Autodesk Fusion 360 part; units mm, degrees
sketch "草图1" plane through (0, 0, 0) normal (0, 1, 0) x (1, 0, 0)
  circle A0 centre (0, 0) radius 10
  circle A1 centre (0, 0) radius 8
  dimension "d1" = 2
extrude "拉伸1" add sketch "草图1" along normal blind 3 contours A1 makes body 1
extrude "拉伸2" add sketch "草图1" along normal blind 5 separate body makes body 2
cylinder "圆柱体基本要素1" add diameter 2 height 20 placed x (1, 0, 0) y (0, 0, -1) z (0, 1, 0) at (20, 0, 1) separate body makes body 3
move_body "对齐1" bodies 3 to x (1, 0, 0) y (0, 1, 0) z (0, 0, 1) at (-20, 0, -1)
pattern_linear "R-阵列1" count 2 spacing 6 along (0, 0, 1) count 2 spacing 4 along (1, 0, 0) of bodies 3 makes body 4 at (4.995, 13.3333, 0.0996) makes body 5 at (0.995, 13.3333, 6.0996) makes body 6 at (4.995, 13.3333, 6.0996)
move_body "移动1" bodies 3 4 5 6 to x (1, 0, 0) y (0, 1, 0) z (0, 0, 1) at (-1.9322, 0, -3.0915)
combine "合并1" operation cut target body 1 tool bodies 3 4 5 6
combine "合并2" operation add target body 2 tool bodies 1
CAD build for the part. Positions are in the model's coordinates, mm. A direction names the side the tool comes from. Round coordinates to 2 decimals unless told otherwise and drop trailing zeros. Loops run counter-clockwise (first coordinate to the right, second up) from the corner with the lowest first, then second, coordinate; pieces in that order, holes last. Notation, with made-up numbers: (55.25, -22) - (76.25, -22) arc R26 ccw to (76.25, 7) - close; hole circle Ø2 at (-3.5, -24). An arc over 180 degrees is marked (long way). Return JSON: item names as keys, results as strings. Group by question number.
Q1. Band-saw the part on D-D on x = 4.25. Give the cut face in (y, z), plus the area to 3 significant figures.
Q2. Tool access for faces 5 (the face through (-0.978, 1.521, -3.392)), 6 (the face through (-1.73, 3.99, -7.81)): list every direction of +Z, -Z, +X, -X, +Y, -Y with a clear straight run to the whole face (end or side of a thin tool).
Q3. Two-plate mould, pull along X, no slides. Class faces 1 (the face through (0, 0, 0)), 2 (the face through (3.022, 1.521, -3.392)), 3 (the face through (-2.17, 2.46, -9.76)), 4 (the face through (-1.471, 1.521, 3.796)): +X half, -X half, draft (parallel to the pull), parting line (faces both ways), or undercut.
Q4. Band-saw the part on A-A on z = 0. Give the cut face in (x, y), plus the area to 3 significant figures.
Q5. Band-saw the part on C-C on y = 3.25. Give the cut face in (x, z), plus the area to 3 significant figures.
Q6. Band-saw the part on B-B on x = -1.5. Give the cut face in (y, z), plus the area to 3 significant figures.
Q7. Flat gauge pins, fed straight in: pin 1 Ø1.5 at (y, z) = (0.5, 1.5) entering from +X; pin 2 Ø2.5 at (x, z) = (2.07, 2.91) entering from +Y; pin 3 Ø1 at (y, z) = (3, -7) entering from -X. Where does each tip first touch, or does it go through?
Q8. Drill centre lines: line 1 along Z through (x, y) = (1.25, 1.85); line 2 along Z through (x, y) = (0, 3.95); line 3 along Z through (x, y) = (-2.75, 2.3). Where is each one in solid material? Low to high. Write a range as [from, to].
Solutions:
{
 "1": {"outline": "(0, -9.05) - (5, -9.05) - (5, -6.78) - (3, -6.78) - (3, 6.78) - (5, 6.78) - (5, 9.05) - (0, 9.05) - close", "area": "63.4 mm^2"},
 "2": {"face 5": "+Y, -Y", "face 6": "+Y"},
 "3": {"face 1": "draft", "face 2": "undercut", "face 3": "parting line", "face 4": "undercut"},
 "4": {"outline": "(-10, 0) - (10, 0) - (10, 5) - (8, 5) - (8, 3) - (-8, 3) - (-8, 5) - (-10, 5) - close", "area": "68.0 mm^2"},
 "5": {"outline": "circle Ø20 at (0, 0); hole circle Ø16 at (0, 0)", "area": "113 mm^2"},
 "6": {"outline": "(0, -9.89) - (5, -9.89) - (5, -7.86) - (3, -7.86) - (3, -3.99) - (0, -3.99) - close; (0, -2.19) - (3, -2.19) - (3, 2.01) - (0, 2.01) - close; (0, 3.81) - (3, 3.81) - (3, 7.86) - (5, 7.86) - (5, 9.89) - (0, 9.89) - close", "area": "56.6 mm^2"},
 "7": {"pin 1": "stops at x = 9.97", "pin 2": "stops at y = 3", "pin 3": "stops at x = -7.6"},
 "8": {"line 1": "z = [-9.92, -3.67], [-2.52, 2.33], [3.48, 9.92]", "line 2": "z = [-10, -8], [8, 10]", "line 3": "z = [-9.61, -3.67], [-2.52, 2.33], [3.48, 9.61]"}
}
